from build123d import *

# Parameters (mm, degrees)
SKETCH1_R                       = 2
BOSS_EXTRUDE1_DEPTH             = 4.75
CUT_EXTRUDE1_DEPTH              = 2
BOSS_EXTRUDE2_REACH             = 69.423
BOSS_EXTRUDE2_DIRECTION_2_REACH = 69.423
CUT_EXTRUDE2_DEPTH              = 2


with BuildPart() as part:
    # Sketch1 → Boss-Extrude1 (new, symmetric)
    with BuildSketch(Plane(origin=(0, 0, 0), x_dir=(1, 0, 0), z_dir=(0, 1, 0))):
        with BuildLine():
            Line((0, -10.500399217), (-55.93053828, -10.500399217))
            ThreePointArc((-55.93053828, -10.500399217), (-66.430937497, 0), (-55.93053828, 10.500399217))
            Line((-55.93053828, 10.500399217), (0, 10.500399217))
            ThreePointArc((0, 10.500399217), (10.500399217, 0), (0, -10.500399217))
        make_face()
        with Locations(Location((0, 0, 0), (0, 0, 270))):
            Circle(SKETCH1_R, mode=Mode.SUBTRACT)
        with Locations(Location((-55.93053828, 0, 0), (0, 0, 270))):
            Circle(SKETCH1_R, mode=Mode.SUBTRACT)
    extrude(amount=BOSS_EXTRUDE1_DEPTH, both=True)

    # Sketch3 → Cut-Extrude1 (cut, symmetric)
    with BuildSketch(Plane(origin=(0, 0, 0), x_dir=(1, 0, 0), z_dir=(0, 1, 0))):
        with BuildLine():
            Line((-35.751827911, 18.875253657), (-39.299525946, 5.868950542))
            Line((-39.299525946, 5.868950542), (26.645239155, -41.810424095))
            ThreePointArc((26.645239155, -41.810424095), (-18.563858299, -45.972421055), (-48.206523525, -11.584965354))
            Line((-48.206523525, -11.584965354), (-43.887265107, 4.249974277))
            Line((-43.887265107, 4.249974277), (-54.812276631, 12.148974547))
            ThreePointArc((-54.812276631, 12.148974547), (-46.585078234, 19.204535889), (-35.751827911, 18.875253657))
        make_face()
    extrude(amount=CUT_EXTRUDE1_DEPTH, both=True, mode=Mode.SUBTRACT)

    # Boss-Extrude2: up to this face of the body (flat: up to its plane)
    boss_extrude2_end = Plane(part.part.faces().sort_by_distance((-27.96526914, 4.75, 0))[0])
    # Sketch5 → Boss-Extrude2 (add, up to the picked face)
    with BuildSketch(Plane(origin=(0, 0, 0), x_dir=(1, 0, 0), z_dir=(0, 1, 0)), mode=Mode.PRIVATE) as boss_extrude2_sk1:
        with BuildLine():
            ThreePointArc((-24.917700351, 10.500399217), (-40.424119316, 19.553005923), (-55.93053828, 10.500399217))
            Line((-55.93053828, 10.500399217), (-24.917700351, 10.500399217))
        make_face()
    boss_extrude2_tool1 = split(extrude(boss_extrude2_sk1.sketch, amount=BOSS_EXTRUDE2_REACH, mode=Mode.PRIVATE), bisect_by=boss_extrude2_end, keep=Keep.BOTH, mode=Mode.PRIVATE)
    add(boss_extrude2_tool1.solids().sort_by(Axis((-40.424119, 0, -14.214125), (0, 1, 0)))[0])

    # Boss-Extrude2 direction 2: up to this face of the body (flat: up to its plane)
    boss_extrude2_direction_2_end = Plane(part.part.faces().sort_by_distance((-27.96526914, -4.75, 0))[0])
    # Sketch5 → Boss-Extrude2 direction 2 (add, up to the picked face)
    with BuildSketch(Plane(origin=(0, 0, 0), x_dir=(1, 0, 0), z_dir=(0, 1, 0)), mode=Mode.PRIVATE) as boss_extrude2_direction_2_sk1:
        with BuildLine():
            ThreePointArc((-24.917700351, 10.500399217), (-40.424119316, 19.553005923), (-55.93053828, 10.500399217))
            Line((-55.93053828, 10.500399217), (-24.917700351, 10.500399217))
        make_face()
    boss_extrude2_direction_2_tool1 = split(extrude(boss_extrude2_direction_2_sk1.sketch, amount=-BOSS_EXTRUDE2_DIRECTION_2_REACH, mode=Mode.PRIVATE), bisect_by=boss_extrude2_direction_2_end, keep=Keep.BOTH, mode=Mode.PRIVATE)
    add(boss_extrude2_direction_2_tool1.solids().sort_by(Axis((-40.424119, 0, -14.214125), (0, -1, 0)))[0])

    # Sketch6 → Cut-Extrude2 (cut, symmetric)
    with BuildSketch(Plane(origin=(0, 0, 0), x_dir=(1, 0, 0), z_dir=(0, 1, 0))):
        with BuildLine():
            Line((-39.299525946, 5.868950542), (-16.659276721, -10.500399217))
            Line((-16.659276721, -10.500399217), (-47.910689027, -10.500399217))
            Line((-47.910689027, -10.500399217), (-43.887265107, 4.249974277))
            Line((-43.887265107, 4.249974277), (-54.854382526, 12.179417945))
            ThreePointArc((-54.854382526, 12.179417945), (-46.349897212, 18.538096729), (-35.738154791, 18.925381021))
            Line((-35.738154791, 18.925381021), (-39.299525946, 5.868950542))
        make_face()
    extrude(amount=CUT_EXTRUDE2_DEPTH, both=True, mode=Mode.SUBTRACT)


solid = part.part
Input: part model. Units: mm. Frame: model coordinates. A direction names the side the tool comes from. Coordinates: 2 decimals unless noted, no trailing zeros. Order: outer loops, then holes, each group sorted by start corner. A loop starts at its lowest first (then second) coordinate and runs counter-clockwise, first axis right, second up. Notation, with made-up numbers: M 51,0 L 61,0 A11 cw 61,14 Z; hole C -24,-27.5 d3. An arc over 180 degrees is marked long. One line per question, with ' | ' between items.
Item 1: Section A-A (z = 0). Output: boundary loops of the cut face in (x, y).
Geometry results:
outline: M -66.43,-4.75 L -57.93,-4.75 L -57.93,4.75 L -66.43,4.75 Z; M -53.93,-4.75 L -2,-4.75 L -2,4.75 L -53.93,4.75 Z; M 2,-4.75 L 10.5,-4.75 L 10.5,4.75 L 2,4.75 Z; hole M -45.05,-2 L -31.18,-2 L -31.18,2 L -45.05,2 Z
Item 2: Section C-C (z = 5). Output: boundary loops of the cut face in (x, y), then the cut area to 3 significant figures.
Geometry results:
outline: M -65.16,-4.75 L 9.23,-4.75 L 9.23,4.75 L -65.16,4.75 Z; hole M -46.41,-2 L -24.27,-2 L -24.27,2 L -46.41,2 Z | area: 618 mm^2
Item 3: Section D-D (x = -24). Output: boundary loops of the cut face in (y, z), then the cut area to 3 significant figures.
Geometry results:
outline: M -4.75,-10.5 L 4.75,-10.5 L 4.75,10.5 L 2,10.5 L 2,5.19 L -2,5.19 L -2,10.5 L -4.75,10.5 Z | area: 178 mm^2
Item 4: Section B-B (y = 4). Output: boundary loops of the cut face in (x, z).
Geometry results:
outline: M -55.93,-10.5 A17.81 ccw -24.92,-10.5 L 0,-10.5 A10.5 ccw 0,10.5 L -55.93,10.5 A10.5 ccw Z; hole C -55.93,0 d4; hole C 0,0 d4
Item 5: Reachability of faces 4 (the flat face through (-28.14, 0.03, 2.2)), 5 (the flat face through (-13, 0, -10.5)), 6 (the flat face through (-40, 2, -1)) from +Z, -Z, +X, -X, +Y, -Y: full face, straight path, thin tool, end or side. Return the list, or none.
Geometry results:
face 4: +Z | face 5: -Z, +X, +Y, -Y | face 6: none
Item 6: Ray query, line 1 along X through (y, z) = (1, 0); line 2 along X through (y, z) = (1, -3); line 3 along Z through (x, y) = (-1.5, 4.25). Return the intervals inside material, ascending.
Geometry results:
line 1: x = -66.43 to -57.93, -53.93 to -45.05, -31.18 to -2, 2 to 10.5 | line 2: x = -65.99 to -44.23, -35.33 to 10.06 | line 3: z = -10.5 to -1.32, 1.32 to 10.5
Item 7: Pin query (flat end, axial travel): pin 1 (3 mm diameter, centred on x = -51, y = 1, fed in from -Z); pin 2 (3 mm diameter, centred on x = -38, y = 0, fed in from +Z); pin 3 (5 mm diameter, centred on y = 1, z = -8, fed in from +X). Return the tip coordinate at first contact, or that it passes through.
Geometry results:
pin 1: stops at z = -16.83 | pin 2: stops at z = -3.84 | pin 3: stops at x = 8.94
Item 8: Draft query along Y for faces 1 (the flat face through (-45.927, 0.028, 3.228)), 2 (the flat face through (-27, 4.75, -1)), 3 (the cylindrical face through (10.5, 0.1, -0.2)). Return one class per face: released by +Y, released by -Y, zero draft, split by the parting line, or undercut.
Geometry results:
face 1: undercut | face 2: released by +Y | face 3: zero draft
